Autodesk Inventor part; units mm, degrees
ref_plane "YZ Plane" through (0, 0, 0) normal (1, 0, 0) x (0, 1, 0)
ref_plane "XZ Plane" through (0, 0, 0) normal (0, 1, 0) x (-1, 0, 0)
ref_plane "XY Plane" through (0, 0, 0) normal (0, 0, 1) x (1, 0, 0)
sketch "Sketch1" plane through (0, 0, 0) normal (0, 0, 1) x (1, 0, 0)
  line L0 (0, 0) -> (0, 22.1615) construction
  line L1 (-11.176, 22.1615) -> (-11.176, 0)
  line L2 (-11.176, 0) -> (-17.526, 0)
  line L3 (-17.526, 0) -> (-17.526, 1.5875)
  line L4 (-17.526, 1.5875) -> (-47.625, 1.5875)
  line L5 (-47.625, 1.5875) -> (-47.625, 14.2875)
  line L6 (-47.625, 14.2875) -> (-19.05, 14.2875)
  line L7 (-33.274, 14.2875) -> (-33.274, 1.5875) construction
  line L8 (-11.176, 22.1615) -> (-19.05, 22.1615)
  line L9 (-19.05, 22.1615) -> (-19.05, 14.2875)
  dimension "SB" = 22.352
  dimension "d1" = 1.5875
  dimension "SL" = 20.574
  dimension "Thickness" = 12.7
  dimension "R" = 35.052
  dimension "OD" = 95.25
  dimension "BC" = 66.548
  dimension "HB" = 38.1
revolve "Revolution1" add sketch "Sketch1" angle 360 about axis through (0, 0, 0) along (0, 1, 0)
sketch "Sketch2" plane through (0, 14.2875, 0) normal (0, 1, 0) x (1, 0, 0)
  line L0 (0, 0) -> (0, 47.625) construction
  circle A0 centre (0, 0) radius 47.625
  line L1 (0, 0) -> (23.5283, 23.5283) construction
  dimension "d11" = 45
  dimension "d12" = 33.274
hole "Hole1" at (23.5283, 14.2875, -23.5283) direction (0, -1, 0) diameter 16.002 depth 12.7
pattern_circular "Circular Pattern1" count 4 over 360 about axis through (0, -10, 0) along (0, 1, 0) of "Hole1"
equation "\"d12\" = 0.5 * BC"
properties part number "ANSI-B300-0.5S"
Here's how the part is built. I have some questions about the finished solid (model axes, mm). A direction names the side the tool comes from. Round coordinates to 2 decimals unless told otherwise and drop trailing zeros. Loops run counter-clockwise (first coordinate to the right, second up) from the corner with the lowest first, then second, coordinate; pieces in that order, holes last.
1. For P1, Ø2, axis at x = -13, y = 13.5, coming from the +Z side; P2, Ø18.5, axis at x = -23.53, z = 23.53, coming from the +Y side; P3, Ø2, axis at y = 17.5, z = 4.5, coming from the -X side, each with a flat end and sliding along its axis, tell me the tip position at first contact or that it passes through.
Answer list:
P1: stops at z = 46.09
P2: stops at y = 14.29
P3: stops at x = -18.73
2. If we section it at C-C on y = 13: Write out the boundary of the cut face in (x, z) (3 decimals).
Answer list:
outline: circle Ø95.25 at (0, 0); hole circle Ø16.002 at (-23.528, -23.528); hole circle Ø16.002 at (-23.528, 23.528); hole circle Ø22.352 at (0, 0); hole circle Ø16.002 at (23.528, -23.528); hole circle Ø16.002 at (23.528, 23.528)
3. If we section it at D-D on x = 13: Write out the boundary of the cut face in (y, z), plus the area to 3 significant figures.
Answer list:
outline: (0, -11.75) - (1.59, -11.75) - (1.59, -45.82) - (14.29, -45.82) - (14.29, -13.92) - (22.16, -13.92) - (22.16, 13.92) - (14.29, 13.92) - (14.29, 45.82) - (1.59, 45.82) - (1.59, 11.75) - (0, 11.75) - close
area: 1,420 mm2
4. Which directions (+Z, -Z, +X, -X, +Y, -Y) give clear straight access to the entire face, cutting with the end or side of a thin tool? Please do faces 1 (the face through (15.12, 18.17, 11.59)), 2 (the face through (-20, 1.588, 1)), 3 (the face through (-25.26, 7.85, -31.34)).
Answer list:
face 1: +Y
face 2: -Y
face 3: +Y, -Y
5. If I drill on line 1 along X through (y, z) = (10.25, -26.5); line 2 along X through (y, z) = (20.25, -0.5); line 3 along X through (y, z) = (9.75, 27), over which ranges is the centre line in solid material (lowest first)?
Answer list:
line 1: x = -39.57 to -30.96, -16.1 to 16.1, 30.96 to 39.57
line 2: x = -19.04 to -11.16, 11.16 to 19.04
line 3: x = -39.23 to -30.74, -16.32 to 16.32, 30.74 to 39.23
6. We'd pull the mould along Z, two halves only. Please class faces 4 (the face through (-31.34, 7.85, 25.26)), 5 (the face through (-8.2, 22.162, -8.2)), 6 (the face through (-16.72, 0.8, 5.26)): +Z half, -Z half, draft (parallel to the pull), parting line (faces both ways), or undercut.
Answer list:
face 4: undercut
face 5: draft
face 6: parting line
